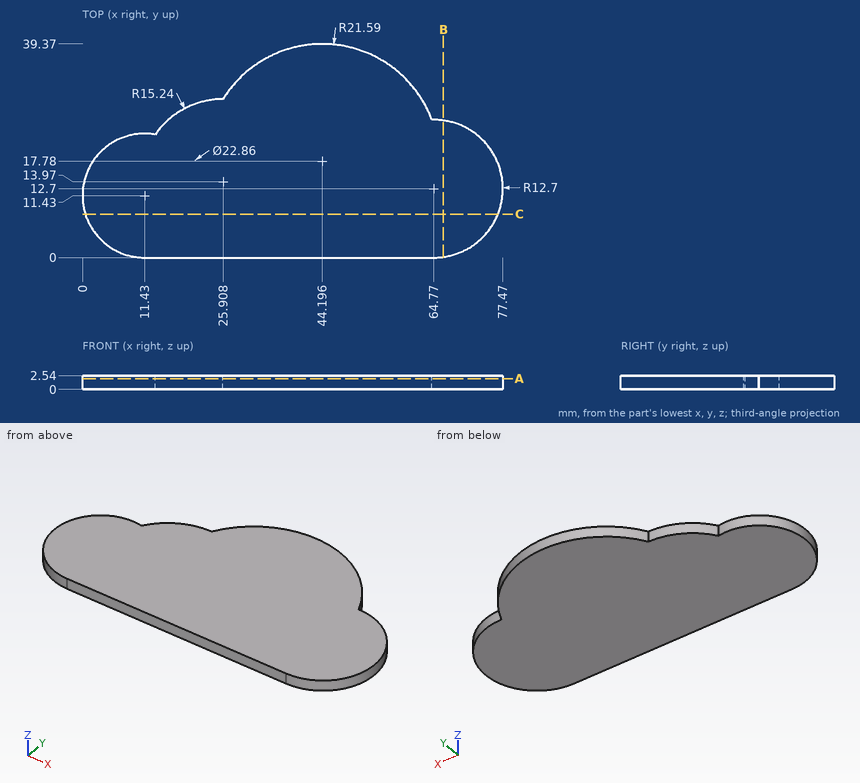
Design review of the part shown in the three views and the two pictorial views. Dimensions are in mm from the part's minimum x, y and z. Round coordinates to 2 decimals unless told otherwise and drop trailing zeros. Loops run counter-clockwise (first coordinate to the right, second up) from the corner with the lowest first, then second, coordinate; pieces in that order, holes last.
1) Consider section C-C on y = 8. State the section outline as (x, z) points, then the cut area to 3 significant figures.
Values follow:
outline: (0.53, 0) - (76.57, 0) - (76.57, 2.54) - (0.53, 2.54) - close
area: 193 mm2
2) Consider section A-A on z = 2. State the section outline as (x, y) points.
Values follow:
outline: (11.43, 0) - (64.77, 0) arc R12.7 ccw (long way) to (64.4, 25.39) arc R21.59 ccw to (25.88, 29.21) arc R15.24 ccw to (13.41, 22.69) arc R11.43 ccw (long way) to start
3) Consider section B-B on x = 66.5. State the section outline as (y, z) points, then the cut area to 3 significant figures.
Values follow:
outline: (0.12, 0) - (25.28, 0) - (25.28, 2.54) - (0.12, 2.54) - close
area: 63.9 mm2
4) Wall thickness on line 1 along X through (y, z) = (4, 0.35); line 2 along X through (y, z) = (35, 1.15); line 3 along Y through (x, z) = (31.5, 0.9): over which ranges is each line inside the solid? List them lowest first.
Values follow:
line 1: x = 2.74 to 74.02
line 2: x = 31.17 to 57.22
line 3: y = 0 to 35.24
